Could you check a few things on this model? Use its own coordinates, in mm. A direction names the side the tool comes from. Coordinates: 2 decimals unless noted, no trailing zeros. Write each loop counter-clockwise with the first axis right and the second up, starting at its lowest first coordinate (ties: lowest second). Pieces come first, ordered by that corner, then holes. Notation, with made-up numbers: M 40.5,71 L 60.5,71 A14 ccw 60.5,85 Z; hole C 31,61.5 d8. An arc over 180 degrees is marked long. Answer as CSV lines item,"result". Start each with the question number.
Item 1: Suppose I cut it at B-B, the plane y = 46.5. Write out the boundary of the cut face in (x, z), and give its area (3 significant figures).
Item 2: On a 3-axis mill with a long thin cutter (end or side, diameter ignored), from which of +Z, -Z, +X, -X, +Y, -Y can I reach the whole of each face in a straight line? I mean faces 4 (the flat face through (10, 203, -1.5)), 5 (the flat face through (10, 400, -1)). Say none if no direction works.
Item 3: Suppose I cut it at A-A, the plane z = -5. Write out the boundary of the cut face in (x, y), and give its area (3 significant figures).
Item 4: I'm going to push a flat-ended pin straight in: P1, Ø5.5, axis at x = 10, y = 200, coming from the -Z side. Where does the tip first touch, or does it pass through?
Item 5: We'd pull the mould along X, two halves only. Please class faces 1 (the flat face through (17.5, 203, -5)), 2 (the flat face through (10, 0, -1)), 3 (the flat face through (20, 197, -4)): +X half, -X half, draft (parallel to the pull), parting line (faces both ways), or undercut.
Item 6: If I drill on line 1 along Y through (x, z) = (10, -0.8); line 2 along X through (y, z) = (173, -4.5); line 3 along X through (y, z) = (385, -0.65), over which ranges is the centre line in solid material (lowest first)? Write a range as [from, to].
```python
from build123d import *

# Parameters (mm, degrees)
SKETCH1_W           = 20
SKETCH1_H           = 8
BOSS_EXTRUDE1_DEPTH = 400
SKETCH2_W           = 15
SKETCH2_H           = 13
CUT_EXTRUDE1_DEPTH  = 401
SKETCH3_R           = 1.75
CUT_EXTRUDE2_DEPTH  = 2.5


with BuildPart() as part:
    # Sketch1 → Boss-Extrude1 (new body)
    with BuildSketch(Plane(origin=(0, 0, 0), x_dir=(1, 0, 0), z_dir=(0, 1, 0))):
        with Locations((10, 4)):
            Rectangle(SKETCH1_W, SKETCH1_H)
    extrude(amount=BOSS_EXTRUDE1_DEPTH)

    # Sketch2 → Cut-Extrude1 (cut, through all)
    with BuildSketch(Plane(origin=(0, 400, 0), x_dir=(1, 0, 0), z_dir=(0, 1, 0))):
        with Locations((10, 8)):
            Rectangle(SKETCH2_W, SKETCH2_H)
    extrude(amount=-CUT_EXTRUDE1_DEPTH, mode=Mode.SUBTRACT)

    # Sketch3 → Cut-Extrude2 (cut, through all)
    with BuildSketch(Plane(origin=(0, 0, -1.5), x_dir=(-1, 0, 0), z_dir=(0, 0, -1))):
        with Locations((-10, 385)):
            Circle(SKETCH3_R)
        with Locations((-10, 200)):
            Circle(SKETCH3_R)
        with Locations((-10, 15)):
            Circle(SKETCH3_R)
    extrude(amount=-CUT_EXTRUDE2_DEPTH, mode=Mode.SUBTRACT)


solid = part.part
```
Ans:
1,outline,"M 0,-8 L 2.5,-8 L 2.5,-1.5 L 17.5,-1.5 L 17.5,-8 L 20,-8 L 20,0 L 0,0 Z"
1,area,"62.5 mm^2"
2,face 4,"-Z, +Y, -Y"
2,face 5,"+Z, -Z, +X, -X, +Y"
3,outline,"M 0,0 L 2.5,0 L 2.5,400 L 0,400 Z; M 17.5,0 L 20,0 L 20,400 L 17.5,400 Z"
3,area,"2,000 mm^2"
4,P1,"stops at z = -1.5"
5,face 1,"undercut"
5,face 2,"draft"
5,face 3,"+X half"
6,line 1,"y = [0, 13.25], [16.75, 198.25], [201.75, 383.25], [386.75, 400]"
6,line 2,"x = [0, 2.5], [17.5, 20]"
6,line 3,"x = [0, 8.25], [11.75, 20]"
